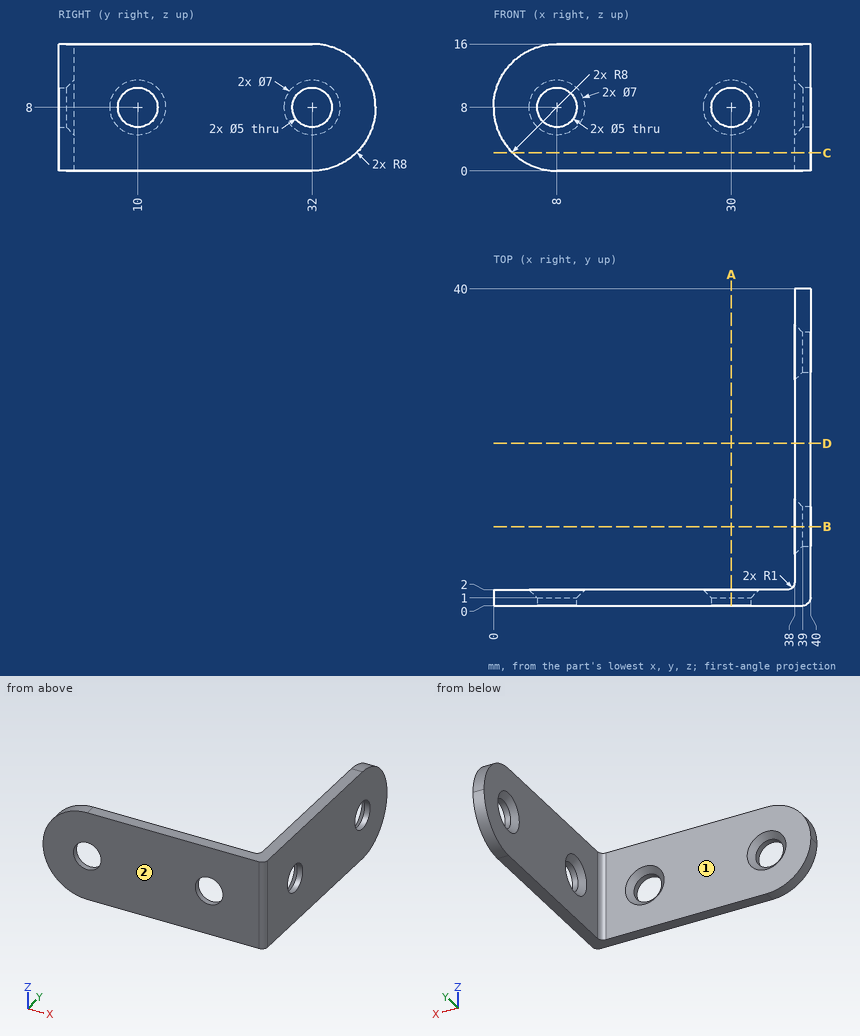
For this review, use the dimensioned drawing (mm, ordinates from the lowest corner) and the shaded views. A direction names the side the tool comes from. Round coordinates to 2 decimals unless told otherwise and drop trailing zeros. Order: outer loops, then holes, each group sorted by start corner. A loop starts at its lowest first (then second) coordinate and runs counter-clockwise, first axis right, second up. Notation, with made-up numbers: (-40, 9) -> (-23, 9) arc R21 ccw to (-23, 18) -> close; hole circle Ø11 at (26.25, 51). An arc over 180 degrees is marked (long way). Write item = value, one per line. Start each with the question number.
Item 1: Clearance check with flat-ended pins moving along their axes: pin 1 Ø6 at (y, z) = (10, 8) entering from -X; pin 2 Ø1 at (x, z) = (17.5, 12) entering from +Y; pin 3 Ø5 at (y, z) = (22.5, 9.5) entering from -X; pin 4 Ø4.5 at (y, z) = (32, 8) entering from -X. State where each tip first meets the part, or that it passes through.
Item 2: For line 1 along Z through (x, y) = (39.65, 10); line 2 along Y through (x, z) = (34.5, 14); line 3 along X through (y, z) = (37.5, 10.25), list the stretches that pass through material, from the lowest coordinate up.
Item 3: Consider section D-D on y = 20.5. Write out the cut boundary in (x, z).
Item 4: Consider section A-A on x = 30. Write out the cut boundary in (y, z), plus the area to 3 significant figures.
Item 5: For the marked faces 1 and 2, list the 3-axis set-ups (+Z, -Z, +X, -X, +Y, -Y) from which the entire face can be reached by the end or side of a thin tool; tool diameter is ignored.
Item 6: Consider section B-B on y = 10. Write out the cut boundary in (x, z).
Item 7: Consider section C-C on z = 2.25. Write out the cut boundary in (x, y).
Conclusion:
q1.pin_1 = 38.5
q1.pin_2 = 2
q1.pin_3 = 38
q1.pin_4 = through
q2.line_1 = 0 to 5.5, 10.5 to 16
q2.line_2 = 0 to 2
q2.line_3 = 38 to 40
q3.outline = (38, 0) -> (40, 0) -> (40, 16) -> (38, 16) -> close
q4.outline = (0, 0) -> (2, 0) -> (2, 4.5) -> (1, 5.5) -> (0, 5.5) -> close; (0, 10.5) -> (1, 10.5) -> (2, 11.5) -> (2, 16) -> (0, 16) -> close
q4.area = 21.0 mm2
q5.face_1 = +Z, -Z, -X, +Y
q5.face_2 = +Z, -Z, +X, -X, -Y
q6.outline = (38, 0) -> (40, 0) -> (40, 5.5) -> (39, 5.5) -> (38, 4.5) -> close; (38, 11.5) -> (39, 10.5) -> (40, 10.5) -> (40, 16) -> (38, 16) -> close
q7.outline = (2.44, 0) -> (39, 0) arc R1 ccw to (40, 1) -> (40, 37.56) -> (38, 37.56) -> (38, 3) arc R1 cw to (37, 2) -> (2.44, 2) -> close
